The model under review builds one solid part; all positions refer to its coordinate system, in mm. Coordinates: 2 decimals unless noted, no trailing zeros. Loops run counter-clockwise (first coordinate to the right, second up) from the corner with the lowest first, then second, coordinate; pieces in that order, holes last. Notation, with made-up numbers: M 28,37 L 42,37 A18 cw 42,57 Z; hole C 25,69.25 d10. An arc over 180 degrees is marked long. Write item = value, one per line. Start each with the question number.
Q1. Clearance check with flat-ended pins moving along their axes: pin 1 Ø4.5 at (x, y) = (69.5, 4.59) entering from -Z; pin 2 Ø4 at (x, y) = (175, -25.75) entering from +Z; pin 3 Ø0.7 at (y, z) = (6, 0.5) entering from -X; pin 4 Ø0.7 at (x, z) = (30, 0.5) entering from +Y. State where each tip first meets the part, or that it passes through.
Q2. Wall thickness on probe 1 along X at (y, z) = (-18, 1.2) (3 decimals); probe 2 along Y at (x, z) = (64.05, 0.2); probe 3 along Y at (x, z) = (89, 0.15): over which ranges is each line inside the solid? List them lowest first.
Q3. We need section A-A on x = 97. Give the boundary of the cut face in (y, z).
Q4. We need section C-C on z = 0.75. Count the separate pieces of the cut face and the enclosed holes in it, and give its area (3 significant figures).
Q5. We need section B-B on x = 69.5. Give the boundary of the cut face in (y, z).
Autodesk Inventor part; units mm, degrees
ref_plane "YZ Plane" through (0, 0, 0) normal (1, 0, 0) x (0, 1, 0)
ref_plane "XZ Plane" through (0, 0, 0) normal (0, 1, 0) x (-1, 0, 0)
ref_plane "XY Plane" through (0, 0, 0) normal (0, 0, 1) x (1, 0, 0)
ref_plane "Work Plane1" through (0, 0, 0) normal (0, 0, 1) x (1, 0, 0)
ref_plane "Work Plane2" through (0, 0, 0) normal (0, 0, 1) x (1, 0, 0)
sketch "Sketch3" plane through (0, 0, 0) normal (0, 0, 1) x (1, 0, 0)
  circle A0 centre (3, -25.75) radius 2.3
  circle A1 centre (3, -3) radius 2.3
  circle A2 centre (3, -74.8889) radius 2.3
  line L0 (0, 0) -> (6, 0)
  line L1 (0, -77.8889) -> (0, 0)
  line L2 (0, -77.8889) -> (6, -77.8889)
  line L3 (6, -71.8889) -> (6, -77.8889)
  line L4 (6, -71.8889) -> (1.6, -71.8889)
  line L5 (1.6, -71.8889) -> (1.6, -56.7889)
  line L6 (1.6, -56.7889) -> (3, -56.7889)
  line L7 (3, -28.75) -> (3, -56.7889)
  line L8 (3, -28.75) -> (6, -28.75)
  line L9 (6, -28.75) -> (6, -22.75)
  line L10 (6, -22.75) -> (3, -22.75)
  line L11 (3, -6) -> (3, -22.75)
  line L12 (3, -6) -> (6, -6)
  line L13 (6, -6) -> (6, 0)
  circle A3 centre (175, -3) radius 2.3
  circle A4 centre (175, -25.75) radius 2.3
  line L14 (175, -28.75) -> (175, -71.8889)
  line L15 (175, -6) -> (175, -22.75)
  line L16 (172, -71.8889) -> (172, -77.8889)
  line L17 (178, -77.8889) -> (172, -77.8889)
  line L18 (178, -77.8889) -> (178, 0)
  line L19 (178, 0) -> (172, 0)
  line L20 (172, 0) -> (172, -6)
  line L21 (172, -6) -> (175, -6)
  line L22 (175, -22.75) -> (172, -22.75)
  line L23 (172, -22.75) -> (172, -28.75)
  line L24 (172, -28.75) -> (175, -28.75)
  circle A5 centre (175, -74.8889) radius 2.3
  circle A6 centre (89, 0.9661) radius 2.3
  circle A7 centre (89, 29.5) radius 2.3
  circle A8 centre (89, 15.55) radius 3.3
  circle A9 centre (89, -14.375) radius 3.3
  circle A10 centre (89, 41.2) radius 3.3
  line L25 (93.5, -27.75) -> (84.5, -27.75)
  line L26 (93.5, 55) -> (93.5, -27.75)
  line L27 (84.5, 55) -> (93.5, 55)
  line L28 (84.5, -27.75) -> (84.5, 55)
  line L29 (105.5, -27.75) -> (111.5, -27.75)
  line L30 (111.5, -24.9105) -> (111.5, -27.75)
  arc A11 (105.5, -24.9105) -> (111.5, -24.9105) centre (108.5, -23.95) ccw
  line L31 (105.5, -27.75) -> (105.5, -24.9105)
  arc A12 (111.5, -22.9895) -> (105.5, -22.9895) centre (108.5, -23.95) ccw
  line L32 (111.5, -5.5855) -> (111.5, -22.9895)
  arc A13 (105.5, -5.5855) -> (111.5, -5.5855) centre (108.5, -4.625) ccw
  line L33 (105.5, -22.9895) -> (105.5, -5.5855)
  circle A14 centre (108.4846, 4.5875) radius 2.3
  arc A15 (105.5, 12.8395) -> (111.5, 12.8395) centre (108.5, 13.8) ccw
  line L34 (105.5, -3.6645) -> (105.5, 12.8395)
  arc A16 (111.5, -3.6645) -> (105.5, -3.6645) centre (108.5, -4.625) ccw
  line L35 (111.5, 12.8395) -> (111.5, -3.6645)
  circle A17 centre (108.4462, 27.5) radius 2.3
  arc A18 (111.5, 14.7605) -> (105.5, 14.7605) centre (108.5, 13.8) ccw
  line L36 (111.5, 40.6331) -> (111.5, 14.7605)
  arc A19 (105.5, 40.1338) -> (111.5, 40.6331) centre (108.4231, 41.3077) ccw
  line L37 (105.5, 14.7605) -> (105.5, 40.1338)
  arc A20 (111.5, 41.9823) -> (105.5, 42.4816) centre (108.4231, 41.3077) ccw
  line L38 (111.5, 55) -> (111.5, 41.9823)
  line L39 (105.5, 55) -> (111.5, 55)
  line L40 (105.5, 42.4816) -> (105.5, 55)
  line L41 (111.5, 41.9823) -> (111.5, 55)
  line L42 (111.5, 41.9823) -> (112.5, 41.9823)
  line L43 (112.5, 41.9823) -> (112.5, 55)
  line L44 (111.5, 55) -> (112.5, 55)
  line L45 (111.5, 14.7605) -> (111.5, 40.6331)
  line L46 (111.5, 14.7605) -> (112.5, 14.7605)
  line L47 (112.5, 14.7605) -> (112.5, 40.6331)
  line L48 (111.5, 40.6331) -> (112.5, 40.6331)
  line L49 (111.5, 0) -> (111.5, 12.8395)
  line L50 (112.5, 0) -> (112.5, 12.8395)
  line L51 (111.5, 12.8395) -> (112.5, 12.8395)
  line L52 (66.5, 14.7605) -> (66.5, 40.6331)
  line L53 (66.5, 40.6331) -> (65.5, 40.6331)
  line L54 (65.5, 14.7605) -> (65.5, 40.6331)
  line L55 (66.5, 14.7605) -> (65.5, 14.7605)
  line L56 (66.5, 41.9823) -> (66.5, 55)
  line L57 (66.5, 55) -> (65.5, 55)
  line L58 (65.5, 41.9823) -> (65.5, 55)
  line L59 (66.5, 41.9823) -> (65.5, 41.9823)
  line L60 (66.5, 0) -> (66.5, 12.8395)
  line L61 (66.5, 12.8395) -> (65.5, 12.8395)
  line L62 (65.5, 0) -> (65.5, 12.8395)
  arc A21 (66.5, -5.5855) -> (72.5, -5.5855) centre (69.5, -4.625) ccw
  line L63 (66.5, -22.9895) -> (66.5, -5.5855)
  arc A22 (72.5, -22.9895) -> (66.5, -22.9895) centre (69.5, -23.95) ccw
  line L64 (72.5, -5.5855) -> (72.5, -22.9895)
  line L65 (66.5, -27.75) -> (72.5, -27.75)
  line L66 (72.5, -24.9105) -> (72.5, -27.75)
  arc A23 (66.5, -24.9105) -> (72.5, -24.9105) centre (69.5, -23.95) ccw
  line L67 (66.5, -27.75) -> (66.5, -24.9105)
  circle A24 centre (69.5, 4.5875) radius 2.3
  arc A25 (72.5, -3.6645) -> (66.5, -3.6645) centre (69.5, -4.625) ccw
  line L68 (72.5, 12.8395) -> (72.5, -3.6645)
  arc A26 (66.5, 12.8395) -> (72.5, 12.8395) centre (69.5, 13.8) ccw
  line L69 (66.5, -3.6645) -> (66.5, 12.8395)
  circle A27 centre (69.5, 27.5) radius 2.3
  arc A28 (66.5, 40.6331) -> (72.5, 40.1338) centre (69.5769, 41.3077) ccw
  line L70 (66.5, 14.7605) -> (66.5, 40.6331)
  arc A29 (72.5, 14.7605) -> (66.5, 14.7605) centre (69.5, 13.8) ccw
  line L71 (72.5, 40.1338) -> (72.5, 14.7605)
  arc A30 (72.5, 42.4816) -> (66.5, 41.9823) centre (69.5769, 41.3077) ccw
  line L72 (72.5, 55) -> (72.5, 42.4816)
  line L73 (66.5, 55) -> (72.5, 55)
  line L74 (66.5, 41.9823) -> (66.5, 55)
  line L75 (56.8, -28.75) -> (56.8, 0)
  line L76 (61.8, -28.75) -> (56.8, -28.75)
  line L77 (61.8, 0) -> (56.8, 0)
  line L78 (61.8, -28.75) -> (66.3, -28.75)
  line L79 (66.3, 0) -> (66.3, -28.75)
  line L80 (61.8, 0) -> (66.3, 0)
  line L81 (116.2, 0) -> (111.7, 0)
  line L82 (111.7, 0) -> (111.7, -28.75)
  line L83 (116.2, -28.75) -> (111.7, -28.75)
  line L84 (121.2, -28.75) -> (121.2, 0)
  line L85 (116.2, 0) -> (121.2, 0)
  line L86 (116.2, -28.75) -> (121.2, -28.75)
  line L87 (0, 0) -> (178, 0)
  line L88 (178, 0) -> (178, -28.75)
  line L89 (178, -28.75) -> (0, -28.75)
  line L90 (0, -28.75) -> (0, 0)
  line L91 (112.5, 0) -> (65.5, 0)
  line L92 (65.5, 0) -> (65.5, 55)
  line L93 (65.5, 55) -> (112.5, 55)
  line L94 (112.5, 55) -> (112.5, 0)
  line L95 (104.5, 11.4325) -> (104.5, -10.5675)
  line L96 (94.5, -10.5675) -> (94.5, 11.4325)
  line L97 (104.5, 11.4325) -> (73.5, 11.4325)
  line L98 (73.5, 11.4325) -> (73.5, -10.5675)
  line L99 (73.5, -10.5675) -> (104.5, -10.5675)
  line L100 (104.5, -10.5675) -> (104.5, 11.4325)
  line L101 (72.5, 12.4325) -> (105.5, 12.4325)
  line L102 (105.5, 12.4325) -> (105.5, -11.5675)
  line L103 (105.5, -11.5675) -> (72.5, -11.5675)
  line L104 (72.5, -11.5675) -> (72.5, 12.4325)
  line L105 (175, -71.8889) -> (172, -71.8889)
  arc A31 (22.05, -4.5875) -> (19.05, -7.5875) centre (22.05, -7.5875) ccw
  line L106 (22.05, -4.5875) -> (43.875, -4.5875)
  line L107 (19.05, -21.225) -> (19.05, -7.5875)
  arc A32 (19.05, -21.225) -> (22.05, -24.225) centre (22.05, -21.225) ccw
  line L108 (43.875, -24.225) -> (22.05, -24.225)
  arc A33 (43.875, -24.225) -> (46.875, -21.225) centre (43.875, -21.225) ccw
  line L109 (46.875, -7.5875) -> (46.875, -21.225)
  arc A34 (46.875, -7.5875) -> (43.875, -4.5875) centre (43.875, -7.5875) ccw
  line L110 (134.125, -4.525) -> (155.95, -4.525)
  arc A35 (158.95, -7.525) -> (155.95, -4.525) centre (155.95, -7.525) ccw
  line L111 (158.95, -7.525) -> (158.95, -21.1625)
  arc A36 (155.95, -24.1625) -> (158.95, -21.1625) centre (155.95, -21.1625) ccw
  line L112 (155.95, -24.1625) -> (134.125, -24.1625)
  arc A37 (131.125, -21.1625) -> (134.125, -24.1625) centre (134.125, -21.1625) ccw
  line L113 (131.125, -21.1625) -> (131.125, -7.525)
  arc A38 (134.125, -4.525) -> (131.125, -7.525) centre (134.125, -7.525) ccw
  line L114 (65.5, 33.8) -> (112.5, 33.8)
  line L115 (66.5, 0) -> (65.5, 0)
  line L116 (111.5, 0) -> (112.5, 0)
  circle A39 centre (64.05, -2.25) radius 1.5
  circle A40 centre (64.05, -26.5) radius 1.5
  circle A41 centre (113.95, -26.5) radius 1.75
  circle A42 centre (113.95, -2.25) radius 1.75
  point P0 (112.5, 0)
  point P1 (65.5, 0)
  point P2 (0, -28.75)
  point P3 (172, 0)
  point P4 (93.5, 12.4325)
  point P5 (105.5, -5.5855)
  point P6 (93.5, -11.5675)
  point P7 (84.5, -11.5675)
  point P8 (72.5, -5.5855)
  point P9 (84.5, 12.4325)
  point P10 (111.5, 33.8)
  dimension "d29" = 1
  dimension "d30" = 1
  dimension "d31" = 1
  dimension "d38" = 4.6
  dimension "d39" = 4.3
extrude "Extrusion2" add sketch "Sketch3" along normal blind 1.4 contours A0 | A1 | L0 L13 L12 L11 L10 L9 L8 L89 L1 | L87 L75 L89 L9 L10 L11 L12 L13 | L77 L80 L79 L78 L76 L75 | L62 L61 L60 L87 L80 | L79 L87 L69 A25 L104 A21 L63 A22 L64 L103 L28 L25 L26 L33 A12 L32 A13 L102 A16 L35 L82 L89 | L92 L55 A29 L71 L114 L28 L101 L68 A26 L61 | L82 L81 L85 L84 L86 L83 | A26 L68 L87 L60 | L54 L114 L52 L55 | L87 L68 A25 L69 | L87 L35 L51 L50 L81 | L52 L114 L71 A29 | L87 L34 A15 L35 | L35 A16 L34 L87 | L84 L87 L20 L21 L15 L22 L23 L89 | L51 A15 L34 L101 L26 L114 L37 A18 L46 L94 | L23 L22 L15 L21 L20 L19 L18 L89 L24 | L101 A8 L26 L97 L28 | L28 L114 L26 L101 A8 | L64 A22 L63 A21 | L87 A6 L26 L99 L28 | L28 L97 L26 L87 A6 | L46 L36 L114 L47 | L101 A8 | A8 L101 | L99 L26 L103 A9 L28 | L87 A6 | A6 L87 | A18 L37 L114 L36 | A13 L32 A12 L33 | L103 A9 L26 L25 L28 | L103 A9 | A9 L103 | A3 | A4 | A7 | L31 A11 L30 L29 | A14 | A17 | L67 A23 L66 L65 | A24 | A27 | A39 | A40 | A41 | A42
sketch "Sketch4" plane through (0, 0, 1.4) normal (0, 0, 1) x (1, 0, 0)
  circle A0 centre (69.5, 27.5) radius 2.3
  circle A1 centre (69.5, 4.5875) radius 2.3
  circle A2 centre (89, 0.9661) radius 2
  circle A3 centre (89, 29.5) radius 2.3
  circle A4 centre (108.4462, 27.5) radius 2.3
  circle A5 centre (108.4846, 4.5875) radius 2.3
  circle A6 centre (3, -25.75) radius 2.3
  circle A7 centre (3, -3) radius 2.3
  circle A8 centre (175, -25.75) radius 2.3
  circle A9 centre (175, -3) radius 2.3
  point P0 (0, 0)
hole "Hole2" at (3, -3, 1.4) at (3, -25.75, 1.4) at (175, -3, 1.4) at (175, -25.75, 1.4) at (108.4846, 4.5875, 1.4) at (89, 0.9661, 1.4) at (69.5, 4.5875, 1.4) at (69.5, 27.5, 1.4) at (89, 29.5, 1.4) at (108.4462, 27.5, 1.4) direction (0, 0, -1) diameter 3.6 end through all countersink diameter 6 countersink angle 90
sketch "Sketch5" plane through (0, 0, 1.4) normal (0, 0, 1) x (1, 0, 0)
  circle A0 centre (64.05, -26.5) radius 1.5
  circle A1 centre (113.95, -26.5) radius 1.5
  circle A2 centre (64.05, -2.25) radius 1.5
  circle A3 centre (113.95, -2.25) radius 1.5
  point P0 (0, 0)
hole "Hole3" at (64.05, -2.25, 1.4) at (64.05, -26.5, 1.4) at (113.95, -26.5, 1.4) at (113.95, -2.25, 1.4) direction (0, 0, -1) diameter 3.1 end through all countersink diameter 5 countersink angle 90
equation "\"d30\" = d29"
properties part number "ceil" material "ABS Plastic"
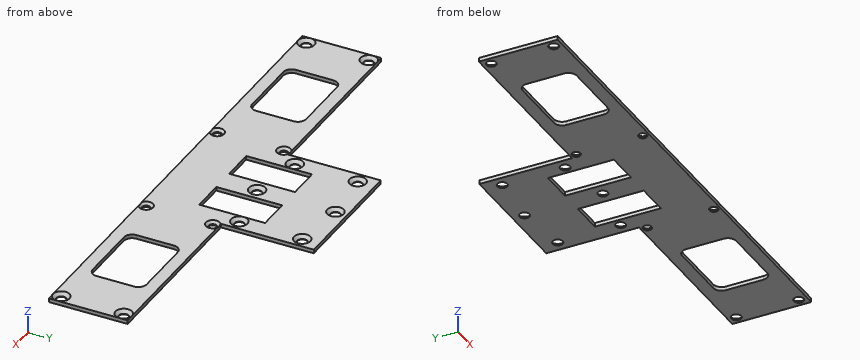
Returned:
q1.pin_1 = 0
q1.pin_2 = 0.4
q1.pin_3 = 65.5
q1.pin_4 = 0
q2.probe_1 = 0 to 19.05, 46.875 to 131.125, 158.95 to 178
q2.probe_2 = -28.75 to -28.05, -24.95 to -3.8, -0.7 to 0
q2.probe_3 = -28.75 to -0.83, 2.77 to 27.7, 31.3 to 33.8
q3.outline = M -28.75,0 L -11.57,0 L -11.57,1.4 L -28.75,1.4 Z; M 12.43,0 L 33.8,0 L 33.8,1.4 L 12.43,1.4 Z
q4.separate_pieces = 1
q4.enclosed_holes = 18
q4.area = 4,840 mm^2
q5.outline = M -28.75,0 L 2.79,0 L 2.79,0.2 L 1.59,1.4 L -28.75,1.4 Z; M 6.39,0 L 25.7,0 L 25.7,0.2 L 24.5,1.4 L 7.59,1.4 L 6.39,0.2 Z; M 29.3,0 L 33.8,0 L 33.8,1.4 L 30.5,1.4 L 29.3,0.2 Z
